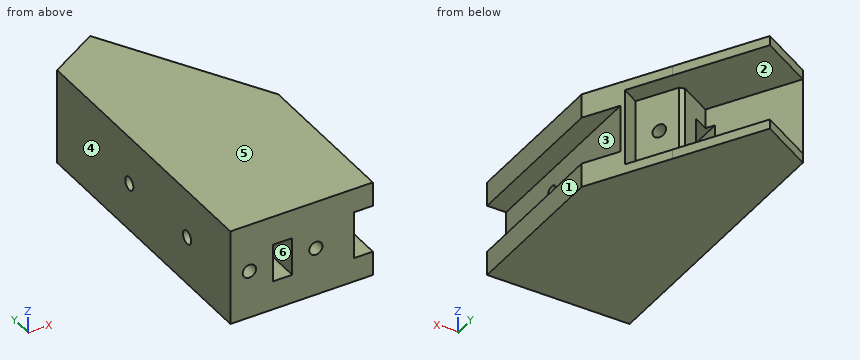
Autodesk Inventor part; units mm, degrees
ref_plane "Work Plane1" through (0, 0, 10.287) normal (0, 0, -1) x (-1, 0, 0)
ref_plane "YZ Plane" through (0, 0, 0) normal (1, 0, 0) x (0, 1, 0)
ref_plane "XZ Plane" through (0, 0, 0) normal (0, 1, 0) x (-1, 0, 0)
sketch "Sketch1" plane through (0, 0, 0) normal (0, 0, 1) x (1, 0, 0)
  line L0 (0, 0) -> (38.1, 0)
  line L1 (38.1, 0) -> (38.1, 41.6033)
  line L2 (0, 76.2) -> (0, 0)
  line L3 (0, 76.2) -> (13.5942, 84.0486)
  line L4 (0, 76.2) -> (12.7, 54.203)
  line L5 (12.7, 54.203) -> (26.2942, 62.0516)
  line L6 (26.2942, 62.0516) -> (13.5942, 84.0486)
  line L7 (26.2942, 62.0516) -> (38.1, 41.6033)
  dimension "d0" = 15.6972
  dimension "d1" = 25.4
  dimension "d2" = 38.1
  dimension "d3" = 76.2
  dimension "d4" = 120
extrude "Extrusion1" add sketch "Sketch1" along normal blind 20.574 contours L2 L4 L5 L7 L1 L0
sketch "Sketch2" plane through (0, 0, 20.574) normal (0, 0, 1) x (1, 0, 0)
  line L0 (0, 76.2) -> (0, 0)
  line L1 (0, 0) -> (38.1, 0)
  line L2 (38.1, 0) -> (38.1, 41.6033)
  line L3 (38.1, 41.6033) -> (26.2942, 62.0516)
  line L4 (26.2942, 62.0516) -> (12.7, 54.203)
  line L5 (12.7, 54.203) -> (0, 76.2)
  line L6 (26.2942, 62.0516) -> (13.5942, 84.0486)
  line L7 (13.5942, 84.0486) -> (0, 76.2)
  line L8 (38.1, 41.6033) -> (26.2942, 62.0516)
extrude "Extrusion2" add sketch "Sketch2" along normal blind 2.54
ref_plane "Work Plane1" through (0, 0, 10.287) normal (0, 0, -1) x (-1, 0, 0)
mirror "Mirror1" about plane through (0, 0, 10.287) normal (0, 0, -1) of "Extrusion2"
sketch "Sketch3" plane through (0, 0, 23.114) normal (0, -1, 0) x (1, 0, 0)
  line L0 (38.1, -25.654) -> (38.1, 0)
  line L1 (38.1, -6.477) -> (33.02, -6.477)
  line L2 (33.02, -6.477) -> (33.02, -19.177)
  line L3 (33.02, -19.177) -> (38.1, -19.177)
  line L4 (38.1, -19.177) -> (38.1, -6.477)
  point P0 (0, -23.114)
  point P1 (38.1, -12.827)
  point P2 (38.1, -19.177)
  dimension "d9" = 12.7
  dimension "d10" = 6.35
  dimension "d11" = 5.08
extrude "Extrusion3" cut sketch "Sketch3" against normal blind 65.0875
sketch "Sketch4" plane through (33.02, 0, 16.637) normal (1, 0, 0) x (0, 0, -1)
  circle A0 centre (6.35, 20.122) radius 1.778
  point P0 (16.637, 0)
extrude "Extrusion4" cut sketch "Sketch4" against normal blind 15.24
sketch "Sketch5" plane through (13.5942, 84.0486, 23.114) normal (0.8660254, 0.5, 0) x (0, 0, -1)
  line L0 (23.114, -25.4) -> (2.54, -25.4)
  line L1 (23.114, -25.4) -> (2.54, -25.4)
  line L2 (2.54, -25.4) -> (2.54, -37.7698)
  line L3 (2.54, -37.7698) -> (23.114, -37.7698)
  line L4 (23.114, -37.7698) -> (23.114, -25.4)
  point P0 (23.114, -65.9911)
  dimension "d16" = 12.3698
extrude "Extrusion5" cut sketch "Sketch5" against normal blind 5.08
chamfer "Chamfer1" distance 1.016 angle 45 1 edges at (21.893, 59.5106, 10.287)
sketch "Sketch6" plane through (9.1948, 81.5086, 23.114) normal (0.8660254, 0.5, 0) x (0, 0, -1)
  line L0 (2.54, -39.2429) -> (2.54, -0.5012)
  line L1 (2.54, -25.4) -> (22.86, -25.4)
  line L2 (23.114, -37.7698) -> (2.54, -37.7698)
  line L3 (2.54, -37.7698) -> (2.54, 0)
  line L4 (2.54, -25.4) -> (2.54, -37.7698)
  circle A0 centre (12.827, -31.5849) radius 1.778
  line L5 (23.114, -37.7698) -> (2.54, -37.7698)
  point P0 (23.114, -65.9911)
  point P1 (2.54, -31.5849)
  point P2 (12.827, -37.7698)
  dimension "d22" = 3.556
extrude "Extrusion6" cut sketch "Sketch6" against normal blind 7.62
ref_plane "Work Plane2" through (0, 0, 10.287) normal (0, 0, 1) x (1, 0, 0)
sketch "Sketch7" plane through (0, 0, 10.287) normal (0, 0, 1) x (1, 0, 0)
  line L0 (21.0149, 59.0036) -> (12.7, 54.203)
  line L1 (16.51, 56.4027) -> (11.43, 56.4027)
  line L2 (12.7, 54.203) -> (0, 76.2)
  line L3 (16.51, 56.4027) -> (16.51, 0)
  line L4 (0, 0) -> (38.1, 0)
  line L5 (11.43, 56.4027) -> (11.43, 0)
  line L6 (11.43, 0) -> (16.51, 0)
  dimension "d25" = 5.08
extrude "Extrusion7" cut sketch "Sketch7" along normal mid plane 10.16 contours L3 L4 L5 L2 L0
sketch "Sketch8" plane through (0, 0, 23.114) normal (-1, 0, 0) x (0, 0, 1)
  circle A0 centre (-12.827, 44.45) radius 1.778
  circle A1 centre (-12.827, 19.05) radius 1.778
  point P0 (-23.114, 0)
extrude "Extrusion8" cut sketch "Sketch8" against normal blind 15.24
sketch "Sketch9" plane through (0, 0, 23.114) normal (0, -1, 0) x (1, 0, 0)
  circle A0 centre (5.08, -12.827) radius 1.778
  circle A1 centre (22.86, -12.827) radius 1.778
  point P0 (0, -23.114)
extrude "Extrusion9" cut sketch "Sketch9" against normal blind 15.24
properties part number "PALM 2"
Input: part model. Units: mm. Frame: model coordinates. Face numbers are marked on the shaded views. A direction names the side the tool comes from. Round coordinates to 2 decimals unless told otherwise and drop trailing zeros. Order: outer loops, then holes, each group sorted by start corner. A loop starts at its lowest first (then second) coordinate and runs counter-clockwise, first axis right, second up. Notation, with made-up numbers: (79, 51.25) - (100, 51.25) arc R12 cw to (100, 70.25) - close; hole circle Ø6 at (-15, -1.5). An arc over 180 degrees is marked (long way). Answer as a JSON object with one key per item and string values. Group by question number.
(1) Reachability of the marked faces 1, 2 and 3 from +Z, -Z, +X, -X, +Y, -Y: full face, straight path, thin tool, end or side. Return the list, or none.
(2) Draft query along Z for the marked faces 4, 5 and 6. Return one class per face: released by +Z, released by -Z, zero draft, split by the parting line, or undercut.
(3) Cut plane C-C (y = 40.5). Return loops of the section in (x, z).
(4) Cut plane A-A (y = 78). Return loops of the section in (x, z), then the cut area to 3 significant figures.
(5) Pin query (flat end, axial travel): P1, Ø12, axis at x = 31, z = 8.5, coming from the +Y side; P2, Ø2, axis at x = 22.5, y = 74, coming from the -Z side; P3, Ø3, axis at y = 20.122, z = 10.287, coming from the +X side; P4, Ø3, axis at x = 12.5, z = 4, coming from the +Y side. Return the tip coordinate at first contact, or that it passes through.
(6) Cut plane D-D (y = 7). Return loops of the section in (x, z).
(7) Material intervals for probe 1 along Z at (x, y) = (14.5, 57); probe 2 along Y at (x, z) = (22, 11); probe 3 along X at (y, z) = (31, 12.75), sorted ascending. Write a range as from..to.
(8) Cut plane B-B (x = 9). Return loops of the section in (y, z) (3 decimals).
Here are the results:
{
 "1": {"face 1": "+Z, -Z, +X, +Y, -Y", "face 2": "+Y", "face 3": "+X, +Y, -Y"},
 "2": {"face 4": "zero draft", "face 5": "released by +Z", "face 6": "undercut"},
 "3": {"outline": "(0, -2.54) - (38.1, -2.54) - (38.1, 3.94) - (33.02, 3.94) - (33.02, 16.64) - (38.1, 16.64) - (38.1, 23.11) - (0, 23.11) - close; hole (11.43, 5.21) - (16.51, 5.21) - (16.51, 15.37) - (11.43, 15.37) - close"},
 "4": {"outline": "(3.12, -2.54) - (17.09, -2.54) - (17.09, 0) - (3.12, 0) - close; (3.12, 20.57) - (17.09, 20.57) - (17.09, 23.11) - (3.12, 23.11) - close", "area": "71.0 mm^2"},
 "5": {"P1": "stops at y = 54.13", "P2": "passes through", "P3": "stops at x = 17.78", "P4": "stops at y = 57.15"},
 "6": {"outline": "(0, -2.54) - (38.1, -2.54) - (38.1, 3.94) - (33.02, 3.94) - (33.02, 16.64) - (38.1, 16.64) - (38.1, 23.11) - (0, 23.11) - close; hole circle Ø3.56 at (5.08, 10.29); hole (11.43, 5.21) - (16.51, 5.21) - (16.51, 15.37) - (11.43, 15.37) - close; hole circle Ø3.56 at (22.86, 10.29)"},
 "7": {"probe 1": "z = -2.54..0, 20.57..23.11", "probe 2": "y = 15.24..18.49, 21.75..50.55, 54.31..58.74", "probe 3": "x = 0..11.43, 16.51..33.02"},
 "8": {"outline": "(0, -2.54) - (81.396, -2.54) - (81.396, 0) - (60.612, 0) - (60.612, 20.574) - (81.396, 20.574) - (81.396, 23.114) - (0, 23.114) - close; hole circle Ø3.556 at (19.05, 10.287); hole circle Ø3.556 at (44.45, 10.287)"}
}
